```python
from build123d import *

# Parameters (mm, degrees)
SKETCH2_W           = 154.686
SKETCH2_H           = 228.6
BOSS_EXTRUDE1_DEPTH = 6.35
SKETCH1_R           = 2.2225
CUT_EXTRUDE1_DEPTH  = 6.35
SKETCH3_W           = 15.24
SKETCH3_H           = 50.8
CUT_EXTRUDE2_DEPTH  = 6.35
SKETCH8_R           = 2.54
CUT_EXTRUDE3_DEPTH  = 17.78


with BuildPart() as part:
    # Sketch2 → Boss-Extrude1 (new body)
    with BuildSketch(Plane(origin=(0, 0, 0), x_dir=(1, 0, 0), z_dir=(0, 1, 0))):
        with Locations((26.543, 26.944051327)):
            Rectangle(SKETCH2_W, SKETCH2_H)
    extrude(amount=BOSS_EXTRUDE1_DEPTH)

    # Sketch1 → Cut-Extrude1 (cut)
    with BuildSketch(Plane(origin=(0, 0, 0), x_dir=(1, 0, 0), z_dir=(0, 1, 0))):
        with Locations((0, 90.444051327)):
            Circle(SKETCH1_R)
        with Locations((53.086, 90.444051327)):
            Circle(SKETCH1_R)
        Circle(SKETCH1_R)
        with Locations((53.086, 0)):
            Circle(SKETCH1_R)
    extrude(amount=CUT_EXTRUDE1_DEPTH, mode=Mode.SUBTRACT)

    # Sketch3 → Cut-Extrude2 (cut)
    with BuildSketch(Plane(origin=(0, 6.35, 0), x_dir=(1, 0, 0), z_dir=(0, 1, 0))):
        with Locations((96.266, 56.154051327)):
            Rectangle(SKETCH3_W, SKETCH3_H)
        with Locations((-43.18, 56.154051327)):
            Rectangle(SKETCH3_W, SKETCH3_H)
    extrude(amount=-CUT_EXTRUDE2_DEPTH, mode=Mode.SUBTRACT)

    # Sketch8 → Cut-Extrude3 (cut)
    with BuildSketch(Plane(origin=(0, 6.35, 0), x_dir=(1, 0, 0), z_dir=(0, 1, 0))):
        with Locations((26.550112, -20.29968)):
            Circle(SKETCH8_R)
        with Locations((-23.077082804, 0.02032)):
            Circle(SKETCH8_R)
        with Locations((76.177306804, 0.02032)):
            Circle(SKETCH8_R)
    extrude(amount=-CUT_EXTRUDE3_DEPTH, mode=Mode.SUBTRACT)


solid = part.part
```
Could you check a few things on this model? Use its own coordinates, in mm. A direction names the side the tool comes from. Round coordinates to 2 decimals unless told otherwise and drop trailing zeros. Loops run counter-clockwise (first coordinate to the right, second up) from the corner with the lowest first, then second, coordinate; pieces in that order, holes last. Notation, with made-up numbers: (20.5, 17) -> (61.5, 17) arc R18 ccw to (61.5, 28) -> close; hole circle Ø5 at (-3.5, 76.25). An arc over 180 degrees is marked (long way). One line per question, with ' | ' between items.
(1) If we section it at C-C on y = 4: List the corners of the cut face in (x, z) for me (1 decimal).
Model answer:
outline: (-50.8, -141.2) -> (103.9, -141.2) -> (103.9, -81.6) -> (88.6, -81.6) -> (88.6, -30.8) -> (103.9, -30.8) -> (103.9, 87.4) -> (-50.8, 87.4) -> (-50.8, -30.8) -> (-35.6, -30.8) -> (-35.6, -81.6) -> (-50.8, -81.6) -> close; hole circle Ø5.1 at (-23.1, 0); hole circle Ø4.4 at (0, -90.4); hole circle Ø4.4 at (0, 0); hole circle Ø5.1 at (26.6, 20.3); hole circle Ø4.4 at (53.1, -90.4); hole circle Ø4.4 at (53.1, 0); hole circle Ø5.1 at (76.2, 0)
(2) For faces 1 (the face through (-43, 3, -81.554)), 2 (the face through (88.646, 3, -56)), 3 (the face through (25, 0, -29)), which set-ups out of +Z, -Z, +X, -X, +Y, -Y let a thin tool reach every point of the face, with its end or its side?
Model answer:
face 1: -X, +Y, -Y | face 2: +X, +Y, -Y | face 3: +Z, -Z, +X, -X, -Y
(3) If we section it at B-B on x = 0: List the corners of the cut face in (y, z) for me.
Model answer:
outline: (0, -141.24) -> (6.35, -141.24) -> (6.35, -92.67) -> (0, -92.67) -> close; (0, -88.22) -> (6.35, -88.22) -> (6.35, -2.22) -> (0, -2.22) -> close; (0, 2.22) -> (6.35, 2.22) -> (6.35, 87.36) -> (0, 87.36) -> close
(4) Thinking about a two-plate mould opening in Z: for faces 4 (the face through (52.604, 3.131, -88.274)), 5 (the face through (25, 6.35, -29)), 6 (the face through (25, 3, -141.244)), which applies, released by +Z, released by -Z, zero draft, split by the parting line, or undercut?
Model answer:
face 4: undercut | face 5: zero draft | face 6: released by -Z
(5) For pin 1 Ø3 at (y, z) = (1.5, -67.5) entering from +X; pin 2 Ø1.9 at (y, z) = (4, -68) entering from -X; pin 3 Ø7 at (x, z) = (53.09, -90.44) entering from -Y, each with a flat end and sliding along its axis, tell me the tip position at first contact or that it passes through.
Model answer:
pin 1: stops at x = 88.65 | pin 2: stops at x = -35.56 | pin 3: stops at y = 0
(6) If I drill on probe 1 along X at (y, z) = (1.5, 0); probe 2 along Z at (x, y) = (0, 2.75); probe 3 along X at (y, z) = (2.5, -65), over which ranges is the centre line in solid material (lowest first)?
Model answer:
probe 1: x = -50.8 to -25.62, -20.54 to -2.22, 2.22 to 50.86, 55.31 to 73.64, 78.72 to 103.89 | probe 2: z = -141.24 to -92.67, -88.22 to -2.22, 2.22 to 87.36 | probe 3: x = -35.56 to 88.65
(7) If we section it at D-D on z = -57: List the corners of the cut face in (x, y) for me.
Model answer:
outline: (-35.56, 0) -> (88.65, 0) -> (88.65, 6.35) -> (-35.56, 6.35) -> close
(8) If we section it at A-A on x = 94.5: List the corners of the cut face in (y, z) for me, and give its area (3 significant figures).
Model answer:
outline: (0, -141.24) -> (6.35, -141.24) -> (6.35, -81.55) -> (0, -81.55) -> close; (0, -30.75) -> (6.35, -30.75) -> (6.35, 87.36) -> (0, 87.36) -> close | area: 1,130 mm^2
